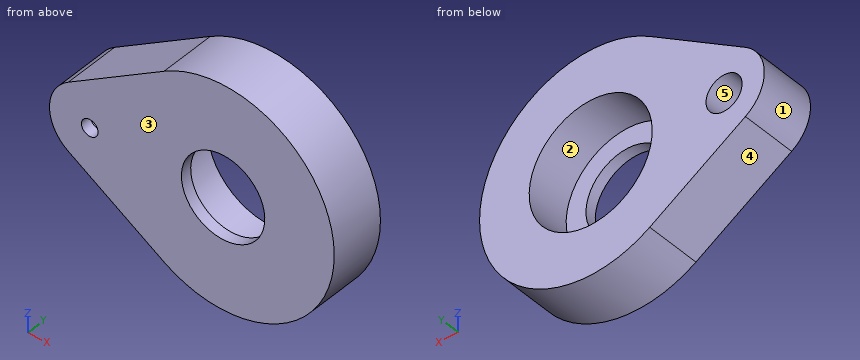
from build123d import *

# Parameters (mm, degrees)
AUFSATZ_LINEAR_AUSTRAGEN1_DEPTH = 10
SKIZZE2_R                       = 3.25
SKIZZE2_R_2                     = 11.075
SCHNITT_LINEAR_AUSTRAGEN1_DEPTH = 8
SKIZZE3_R                       = 7.5
SKIZZE3_R_2                     = 1.5
SCHNITT_LINEAR_AUSTRAGEN2_DEPTH = 2


with BuildPart() as part:
    # Skizze1 → Aufsatz-Linear austragen1 (new body)
    with BuildSketch(Plane(origin=(0, 0, 0), x_dir=(1, 0, 0), z_dir=(0, 1, 0))):
        with BuildLine():
            Line((-3.8515625, -6.142309526), (13.375, -16.94430214))
            ThreePointArc((13.375, -16.94430214), (44, 0), (13.375, 16.94430214))
            Line((13.375, 16.94430214), (-3.8515625, 6.142309526))
            ThreePointArc((-3.8515625, 6.142309526), (-7.25, 0), (-3.8515625, -6.142309526))
        make_face()
    extrude(amount=AUFSATZ_LINEAR_AUSTRAGEN1_DEPTH)

    # Skizze2 → Schnitt-Linear austragen1 (cut)
    with BuildSketch(Plane(origin=(0, 10, 0), x_dir=(1, 0, 0), z_dir=(0, 1, 0))):
        with Locations(Location((0, 0, 0), (0, 0, 270))):
            Circle(SKIZZE2_R)
        with Locations(Location((24, 0, 0), (0, 0, 270))):
            Circle(SKIZZE2_R_2)
    extrude(amount=-SCHNITT_LINEAR_AUSTRAGEN1_DEPTH, mode=Mode.SUBTRACT)

    # Skizze3 → Schnitt-Linear austragen2 (cut)
    with BuildSketch(Plane(origin=(0, 2, 0), x_dir=(1, 0, 0), z_dir=(0, 1, 0))):
        with Locations(Location((24, 0, 0), (0, 0, 270))):
            Circle(SKIZZE3_R)
        with Locations(Location((0, 0, 0), (0, 0, 270))):
            Circle(SKIZZE3_R_2)
    extrude(amount=-SCHNITT_LINEAR_AUSTRAGEN2_DEPTH, mode=Mode.SUBTRACT)


solid = part.part
For this review, take the finished solid that the model builds, in its own axes (mm). Face numbers are marked on the shaded views. A direction names the side the tool comes from. Give positions to 0.01 mm unless a question says otherwise; leave off trailing zeros. Order: outer loops, then holes, each group sorted by start corner. A loop starts at its lowest first (then second) coordinate and runs counter-clockwise, first axis right, second up. Notation, with made-up numbers: (-17.75, 23) - (14.25, 23) arc R13 cw to (14.25, 42) - close; hole circle Ø10 at (19.5, 65). An arc over 180 degrees is marked (long way). Answer as a JSON object with one key per item and string values. Group by question number.
Item 1: Wall thickness on line 1 along X through (y, z) = (6, 0) (3 decimals); line 2 along X through (y, z) = (1.65, 0); line 3 along Y through (x, z) = (16.5, 4): over which ranges is each line inside the solid? List them lowest first.
Item 2: Take a section at A-A on z = 0. Give the boundary of the cut face in (x, y) (3 decimals).
Item 3: Take a section at D-D on z = 9.5. Give the boundary of the cut face in (x, y).
Item 4: Clearance check with flat-ended pins moving along their axes: pin 1 Ø2 at (x, y) = (10.5, 2) entering from +Z; pin 2 Ø2 at (x, z) = (32, 0) entering from -Y; pin 3 Ø6 at (y, z) = (3.5, 11) entering from -X; pin 4 Ø1.8 at (x, z) = (0, 0) entering from +Y. State where each tip first meets the part, or that it passes through.
Item 5: Machinability: for the marked faces 4 and 5, which of the approach directions +Z, -Z, +X, -X, +Y, -Y give a long, thin tool a straight path to every point of the face, cutting with its end or side? Answer none if there is none.
Item 6: Take a section at B-B on x = 24. Give the boundary of the cut face in (y, z) (3 decimals).
Item 7: Draft analysis for pull direction X (two halves, no side actions). For the marked faces 1, 2 and 3, state which applies: pulls with the +X half, pulls with the -X half, needs draft (parallel to the pull), parting line crosses it, or undercut.
Item 8: Take a section at C-C on y = 1. Give the boundary of the cut face in (x, z) (3 decimals), and give its area (3 significant figures).
Reported:
{
 "1": {"line 1": "-7.25 to -3.25, 3.25 to 12.925, 35.075 to 44", "line 2": "-7.25 to -1.5, 1.5 to 16.5, 31.5 to 44", "line 3": "0 to 2"},
 "2": {"outline": "(-7.25, 0) - (-1.5, 0) - (-1.5, 2) - (-3.25, 2) - (-3.25, 10) - (-7.25, 10) - close; (1.5, 0) - (16.5, 0) - (16.5, 2) - (12.925, 2) - (12.925, 10) - (3.25, 10) - (3.25, 2) - (1.5, 2) - close; (31.5, 0) - (44, 0) - (44, 10) - (35.075, 10) - (35.075, 2) - (31.5, 2) - close"},
 "3": {"outline": "(1.5, 0) - (41.6, 0) - (41.6, 10) - (29.69, 10) - (29.69, 2) - (18.31, 2) - (18.31, 10) - (1.5, 10) - close"},
 "4": {"pin 1": "z = 15.77", "pin 2": "y = 0", "pin 3": "x = -0.89", "pin 4": "through"},
 "5": {"face 4": "-Z, -X, +Y, -Y", "face 5": "+Y"},
 "6": {"outline": "(0, -20) - (10, -20) - (10, -11.075) - (2, -11.075) - (2, -7.5) - (0, -7.5) - close; (0, 7.5) - (2, 7.5) - (2, 11.075) - (10, 11.075) - (10, 20) - (0, 20) - close"},
 "7": {"face 1": "pulls with the -X half", "face 2": "undercut", "face 3": "needs draft"},
 "8": {"outline": "(-3.852, -6.142) - (13.375, -16.944) arc R20 ccw (long way) to (13.375, 16.944) - (-3.852, 6.142) arc R7.25 ccw to start; hole circle Ø3 at (0, 0); hole circle Ø15 at (24, 0)", "area": "1,280 mm^2"}
}
